```python
from build123d import *

# Parameters (mm, degrees)
SKETCH1_W           = 44
SKETCH1_H           = 14.5
SKETCH1_W_2         = 40
SKETCH1_H_2         = 10.5
BOSS_EXTRUDE1_DEPTH = 28
SKETCH2_W           = 44
SKETCH2_H           = 14.5
BOSS_EXTRUDE2_DEPTH = 2
CUT_EXTRUDE1_REACH  = 46
SKETCH3_W           = 6
SKETCH3_H           = 12
CUT_EXTRUDE2_REACH  = 46
SKETCH4_W           = 10
SKETCH4_H           = 20


with BuildPart() as part:
    # Sketch1 → Boss-Extrude1 (new body)
    with BuildSketch(Plane(origin=(0, 0, 0), x_dir=(1, 0, 0), z_dir=(0, 1, 0))):
        Rectangle(SKETCH1_W, SKETCH1_H)
        Rectangle(SKETCH1_W_2, SKETCH1_H_2, mode=Mode.SUBTRACT)
    extrude(amount=BOSS_EXTRUDE1_DEPTH)

    # Sketch2 → Boss-Extrude2 (add)
    with BuildSketch(Plane(origin=(0, 0, 0), x_dir=(1, 0, 0), z_dir=(0, 1, 0))):
        Rectangle(SKETCH2_W, SKETCH2_H)
    extrude(amount=-BOSS_EXTRUDE2_DEPTH)

    # Sketch3 → Cut-Extrude1 (cut, up to next)
    with BuildSketch(Plane.ZY.offset(22), mode=Mode.PRIVATE) as cut_extrude1_sk1:
        with Locations((-0.23425331, 14)):
            Rectangle(SKETCH3_W, SKETCH3_H)
    cut_extrude1_tool1 = extrude(cut_extrude1_sk1.sketch, amount=-CUT_EXTRUDE1_REACH, mode=Mode.PRIVATE) & part.part
    add(cut_extrude1_tool1.solids().sort_by_distance((-22, 14, -0.234253))[0], mode=Mode.SUBTRACT)

    # Sketch4 → Cut-Extrude2 (cut, up to next)
    with BuildSketch(Plane(origin=(22, 0, 0), x_dir=(0, 0, -1), z_dir=(1, 0, 0)), mode=Mode.PRIVATE) as cut_extrude2_sk1:
        with Locations((0, 14)):
            Rectangle(SKETCH4_W, SKETCH4_H)
    cut_extrude2_tool1 = extrude(cut_extrude2_sk1.sketch, amount=-CUT_EXTRUDE2_REACH, mode=Mode.PRIVATE) & part.part
    add(cut_extrude2_tool1.solids().sort_by_distance((22, 14, 0))[0], mode=Mode.SUBTRACT)


solid = part.part
```
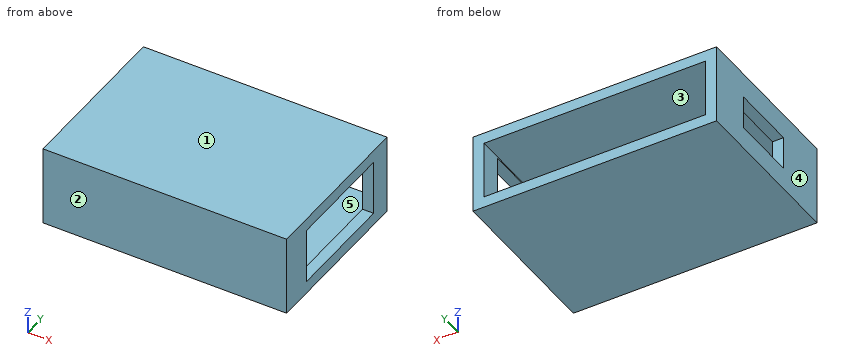
Verification items for the finished model (mm, model axes). Face numbers are marked on the shaded views. A direction names the side the tool comes from. Coordinates: 2 decimals unless noted, no trailing zeros. Loops run counter-clockwise (first coordinate to the right, second up) from the corner with the lowest first, then second, coordinate; pieces in that order, holes last. Notation, with made-up numbers: (26, 86.5) -> (34, 86.5) arc R17 ccw to (34, 106.5) -> close; hole circle Ø10 at (55.25, 54.25). An arc over 180 degrees is marked (long way). Answer in a Markdown table with one row per item. Add a question column.
1. Material ranges on probe 1 along Z at (x, y) = (20.5, 10.5); probe 2 along Z at (x, y) = (6, 14.75); probe 3 along X at (y, z) = (3.5, 0.5), recorded low to high. Write a range as [from, to].
2. Section check C-C, the plane z = 2. Enter the section's corners in (x, y), then the cut area to 3 significant figures.
3. Depth check by flat-ended pin: P1, Ø5, axis at x = 4, z = 2.5, coming from the +Y side. Enter the tip coordinate at first touch or a pass-through.
4. Section check D-D, the plane x = -5. Enter the section's corners in (y, z), then the cut area to 3 significant figures.
5. Access from +Z, -Z, +X, -X, +Y, -Y to the whole of each face (thin tool, end or side, straight path). Record for the marked faces 4 and 5.
6. Section check A-A, the plane z = 4.5. Enter the section's corners in (x, y).
7. Section check B-B, the plane y = 20.5. Enter the section's corners in (x, z).
8. Draft check along Z on the marked faces 1, 2 and 3. Enter one of: +Z half, -Z half, draft (parallel to the pull), parting line (faces both ways), or undercut.
Derived:
| question | item | result |
|---|---|---|
| 1 | probe 1 | z = [-7.25, -5], [5, 7.25] |
| 1 | probe 2 | z = [-7.25, -5.25], [5.25, 7.25] |
| 1 | probe 3 | x = [-22, -20], [20, 22] |
| 2 | outline | (-22, -2) -> (22, -2) -> (22, 4) -> (20, 4) -> (20, 0) -> (-20, 0) -> (-20, 8) -> (-22, 8) -> close; (-22, 20) -> (-20, 20) -> (-20, 28) -> (-22, 28) -> close; (20, 24) -> (22, 24) -> (22, 28) -> (20, 28) -> close |
| 2 | area | 136 mm² |
| 3 | P1 | stops at y = 0 |
| 4 | outline | (-2, -7.25) -> (28, -7.25) -> (28, -5.25) -> (0, -5.25) -> (0, 5.25) -> (28, 5.25) -> (28, 7.25) -> (-2, 7.25) -> close |
| 4 | area | 141 mm² |
| 5 | face 4 | +Z, -Z, -X, +Y, -Y |
| 5 | face 5 | +Y |
| 6 | outline | (-22, -2) -> (22, -2) -> (22, 4) -> (20, 4) -> (20, 0) -> (-20, 0) -> (-20, 28) -> (-22, 28) -> close; (20, 24) -> (22, 24) -> (22, 28) -> (20, 28) -> close |
| 7 | outline | (-22, -7.25) -> (22, -7.25) -> (22, -5) -> (20, -5) -> (20, -5.25) -> (-20, -5.25) -> (-20, 5.25) -> (20, 5.25) -> (20, 5) -> (22, 5) -> (22, 7.25) -> (-22, 7.25) -> close |
| 8 | face 1 | +Z half |
| 8 | face 2 | draft |
| 8 | face 3 | undercut |
